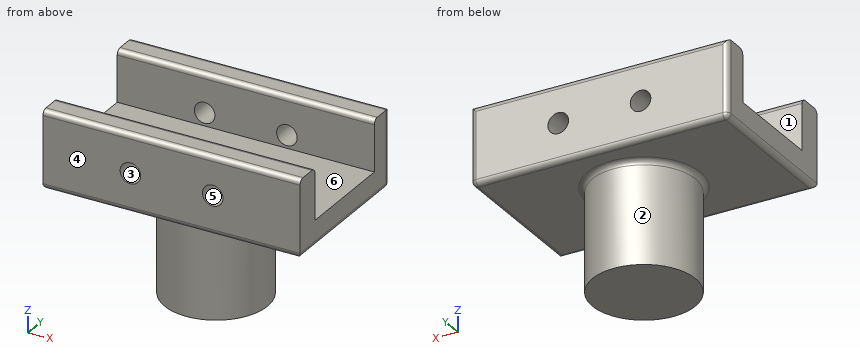
```python
from build123d import *

# Parameters (mm, degrees)
SKETCH1_W           = 50
SKETCH1_H           = 30
BOSS_EXTRUDE1_DEPTH = 15
SKETCH2_W           = 50
SKETCH2_H           = 20
CUT_EXTRUDE1_DEPTH  = 10
SKETCH3_R           = 2
CUT_EXTRUDE2_DEPTH  = 42.833001327
SKETCH4_R           = 10
BOSS_EXTRUDE2_DEPTH = 20
FILLET3_R           = 1
FILLET4_R           = 1
FILLET5_R           = 1
FILLET6_R           = 1
FILLET7_R           = 1


with BuildPart() as part:
    # Sketch1 → Boss-Extrude1 (new body)
    with BuildSketch(Plane.XY):
        Rectangle(SKETCH1_W, SKETCH1_H)
    extrude(amount=BOSS_EXTRUDE1_DEPTH)

    # Sketch2 → Cut-Extrude1 (cut)
    with BuildSketch(Plane.XY.offset(15)):
        Rectangle(SKETCH2_W, SKETCH2_H)
    extrude(amount=-CUT_EXTRUDE1_DEPTH, mode=Mode.SUBTRACT)

    # Sketch3 → Cut-Extrude2 (cut, through all)
    with BuildSketch(Plane(origin=(0, 15, 0), x_dir=(1, 0, 0), z_dir=(0, 1, 0))):
        with Locations(Location((-8, -7.5, 0), (0, 0, 270))):
            Circle(SKETCH3_R)
        with Locations(Location((8, -7.5, 0), (0, 0, 270))):
            Circle(SKETCH3_R)
    extrude(amount=-CUT_EXTRUDE2_DEPTH, mode=Mode.SUBTRACT)

    # Sketch4 → Boss-Extrude2 (add)
    with BuildSketch(Plane(origin=(0, 0, 0), x_dir=(-1, 0, 0), z_dir=(0, 0, -1))):
        Circle(SKETCH4_R)
    extrude(amount=BOSS_EXTRUDE2_DEPTH)

    # Fillet3
    fillet3_edges = [part.edges().sort_by_distance(p)[0] for p in [
        (0, -10, 15),
    ]]
    fillet(fillet3_edges, radius=FILLET3_R)

    # Fillet4
    fillet4_edges = [part.edges().sort_by_distance(p)[0] for p in [
        (0, -15, 15),
    ]]
    fillet(fillet4_edges, radius=FILLET4_R)

    # Fillet5
    fillet5_edges = [part.edges().sort_by_distance(p)[0] for p in [
        (0, -15, 0),
        (-25, 0, 0),
        (0, 15, 0),
        (25, 0, 0),
        (-25, 15, 7.5),
        (25, 15, 7.5),
        (0, 15, 15),
    ]]
    fillet(fillet5_edges, radius=FILLET5_R)

    # Fillet6
    fillet6_edges = [part.edges().sort_by_distance(p)[0] for p in [
        (0, 10, 15),
    ]]
    fillet(fillet6_edges, radius=FILLET6_R)

    # Fillet7
    fillet7_edges = [part.edges().sort_by_distance(p)[0] for p in [
        (10, 0, 0),
    ]]
    fillet(fillet7_edges, radius=FILLET7_R)


solid = part.part
```
Geometry: final body of the model. Coordinates: model frame, mm. Face numbers are marked on the shaded views. A direction names the side the tool comes from. Round coordinates to 2 decimals unless told otherwise and drop trailing zeros. Order: outer loops, then holes, each group sorted by start corner. A loop starts at its lowest first (then second) coordinate and runs counter-clockwise, first axis right, second up. Notation, with made-up numbers: (73, -14) -> (98, -14) arc R28 cw to (98, 15) -> close; hole circle Ø11 at (-10, 21). An arc over 180 degrees is marked (long way). Use one line per item in the form item = value. Start each with the question number.
1. Line query: probe 1 along X at (y, z) = (-12.9, 7.5); probe 2 along Z at (x, y) = (-20, 5.25); probe 3 along Z at (x, y) = (-9.5, -0.5). Output: solid intervals per line, ascending.
2. Pin query (flat end, axial travel): pin 1 Ø10 at (x, y) = (1.5, 7) entering from +Z; pin 2 Ø4 at (y, z) = (7.5, -7.5) entering from +X; pin 3 Ø10 at (x, y) = (-3, -4.5) entering from +Z; pin 4 Ø1 at (x, y) = (10, 11) entering from -Z. Return the tip coordinate at first contact, or that it passes through.
3. Cut plane A-A (z = 7.5). Return the cut outline in (x, y), then the cut area to 3 significant figures.
4. Cut plane C-C (x = 0). Return the cut outline in (y, z), then the cut area to 3 significant figures.
5. Reachability of the marked faces 1, 2 and 3 from +Z, -Z, +X, -X, +Y, -Y: full face, straight path, thin tool, end or side. Return the list, or none.
6. Draft query along Y for the marked faces 4, 5 and 6. Return one class per face: pulls with the +Y half, pulls with the -Y half, needs draft (parallel to the pull), parting line crosses it, or undercut.
7. Cut plane B-B (y = 12.5). Return the cut outline in (x, z).
8. Cut plane D-D (y = 0). Return the cut outline in (x, z), then the cut area to 3 significant figures.
Solution:
q1.probe_1 = -25 to -10, -6 to 6, 10 to 25
q1.probe_2 = 0 to 5
q1.probe_3 = -20 to 5
q2.pin_1 = 15
q2.pin_2 = 8.35
q2.pin_3 = 5
q2.pin_4 = 0
q3.outline = (-25, -15) -> (-10, -15) -> (-10, -10) -> (-25, -10) -> close; (-25, 10) -> (-10, 10) -> (-10, 15) -> (-24, 15) arc R1 ccw to (-25, 14) -> close; (-6, -15) -> (6, -15) -> (6, -10) -> (-6, -10) -> close; (-6, 10) -> (6, 10) -> (6, 15) -> (-6, 15) -> close; (10, -15) -> (25, -15) -> (25, -10) -> (10, -10) -> close; (10, 10) -> (25, 10) -> (25, 14) arc R1 ccw to (24, 15) -> (10, 15) -> close
q3.area = 420 mm^2
q4.outline = (-15, 1) arc R1 ccw to (-14, 0) -> (-11, 0) arc R1 cw to (-10, -1) -> (-10, -20) -> (10, -20) -> (10, -1) arc R1 cw to (11, 0) -> (14, 0) arc R1 ccw to (15, 1) -> (15, 14) arc R1 ccw to (14, 15) -> (11, 15) arc R1 ccw to (10, 14) -> (10, 5) -> (-10, 5) -> (-10, 14) arc R1 ccw to (-11, 15) -> (-14, 15) arc R1 ccw to (-15, 14) -> close
q4.area = 649 mm^2
q5.face_1 = +Z, +X, -X
q5.face_2 = -Z
q5.face_3 = +Y, -Y
q6.face_4 = pulls with the -Y half
q6.face_5 = needs draft
q6.face_6 = undercut
q7.outline = (-25, 1) arc R1 ccw to (-24, 0) -> (24, 0) arc R1 ccw to (25, 1) -> (25, 15) -> (-25, 15) -> close; hole circle Ø4 at (-8, 7.5); hole circle Ø4 at (8, 7.5)
q8.outline = (-25, 1) arc R1 ccw to (-24, 0) -> (-11, 0) arc R1 cw to (-10, -1) -> (-10, -20) -> (10, -20) -> (10, -1) arc R1 cw to (11, 0) -> (24, 0) arc R1 ccw to (25, 1) -> (25, 5) -> (-25, 5) -> close
q8.area = 650 mm^2
